Verification items for the finished model (mm, model axes). Give positions to 0.01 mm unless a question says otherwise; leave off trailing zeros. Loops run counter-clockwise (first coordinate to the right, second up) from the corner with the lowest first, then second, coordinate; pieces in that order, holes last. Notation, with made-up numbers: (6.25, 58) -> (26.25, 58) arc R23 ccw to (26.25, 70) -> close; hole circle Ø6 at (-18.5, 22). An arc over 180 degrees is marked (long way). Use one line per item in the form item = value. Start each with the question number.
from build123d import *

# Parameters (mm, degrees)
SALIENTE_EXTRUIR1_DEPTH = 3


with BuildPart() as part:
    # Croquis1 → Saliente-Extruir1 (new body)
    with BuildSketch(Plane(origin=(0, 0, 0), x_dir=(1, 0, 0), z_dir=(0, 1, 0))):
        with BuildLine():
            Line((0.226595449, 185.804586765), (-22.78, 185.804586765))
            Line((-22.78, 185.804586765), (-22.78, -18.195413235))
            Line((-22.78, -18.195413235), (0, -18.195413235))
            Line((0, -18.195413235), (0, -21.195413235))
            Line((0, -21.195413235), (18.001591933, -21.195413235))
            ThreePointArc((18.001591933, -21.195413235), (18.666950073, -21.163719955), (19.326283246, -21.068927105))
            Line((19.326283246, -21.068927105), (73.612622199, -10.606644927))
            ThreePointArc((73.612622199, -10.606644927), (77.685747073, -8.18998874), (79.287930885, -3.733131057))
            Line((79.287930885, -3.733131057), (79.287930885, 23.819925262))
            ThreePointArc((79.287930885, 23.819925262), (78.94752374, 25.976270087), (77.959410027, 27.922890572))
            Line((77.959410027, 27.922890572), (27.995644059, 96.987197766))
            ThreePointArc((27.995644059, 96.987197766), (26.997710984, 98.702595555), (26.358179585, 100.581281157))
            Line((26.358179585, 100.581281157), (22.262888034, 118.173345099))
            Line((22.262888034, 118.173345099), (7.026156274, 180.467708103))
            ThreePointArc((7.026156274, 180.467708103), (4.548525031, 184.311030689), (0.226595449, 185.804586765))
        make_face()
    extrude(amount=SALIENTE_EXTRUIR1_DEPTH)


solid = part.part
Item 1: Sectioned sample at B-B, the plane z = -42.5. Enter the section's corners in (x, y), and give its area (3 significant figures).
Item 2: Gauge pin test, flat ends, axial feed: pin 1 Ø1 at (y, z) = (1, -141.5) entering from +X; pin 2 Ø1.5 at (y, z) = (1.5, -105.5) entering from +X. Record the tip position at first contact, or that the pin passes through.
Item 3: Material ranges on line 1 (Z direction, x = -18, y = 1.7); line 2 (X direction, y = 1.4, z = -100.5); line 3 (X direction, y = 2.4, z = -121.5), recorded low to high.
Item 4: Sectioned sample at A-A, the plane y = 1.25. Enter the section's corners in (x, z), and give its area (3 significant figures).
Item 5: Sectioned sample at C-C, the plane x = 46. Enter the section's corners in (y, z), and give its area (3 significant figures).
Outcome:
q1.outline = (-22.78, 0) -> (67.41, 0) -> (67.41, 3) -> (-22.78, 3) -> close
q1.area = 271 mm^2
q2.pin_1 = 16.68
q2.pin_2 = 25.39
q3.line_1 = -185.8 to 18.2
q3.line_2 = -22.78 to 26.38
q3.line_3 = -22.78 to 21.45
q4.outline = (-22.78, -185.8) -> (0.23, -185.8) arc R7 ccw to (7.03, -180.47) -> (22.26, -118.17) -> (26.36, -100.58) arc R10 cw to (28, -96.99) -> (77.96, -27.92) arc R7 ccw to (79.29, -23.82) -> (79.29, 3.73) arc R7 ccw to (73.61, 10.61) -> (19.33, 21.07) arc R7 ccw to (18, 21.2) -> (0, 21.2) -> (0, 18.2) -> (-22.78, 18.2) -> close
q4.area = 13,300 mm^2
q5.outline = (0, -72.1) -> (3, -72.1) -> (3, 15.93) -> (0, 15.93) -> close
q5.area = 264 mm^2
